```python
from build123d import *

# Parameters (mm, degrees)
SKETCH1_R         = 15
BODY_DEPTH        = 7
SKETCH2_R         = 11.5
CENTER_HOLE_DEPTH = 18
SKETCH4_W         = 4
SKETCH4_H         = 18.83157123
HEX_2_DEPTH       = 4


with BuildPart() as part:
    # Sketch1 → Body (new body)
    with BuildSketch(Plane(origin=(0, 0, 0), x_dir=(1, 0, 0), z_dir=(0, 1, 0))):
        Circle(SKETCH1_R)
    extrude(amount=BODY_DEPTH)

    # Sketch2 → Center_hole (cut)
    with BuildSketch(Plane(origin=(0, 7, 0), x_dir=(1, 0, 0), z_dir=(0, 1, 0))):
        Circle(SKETCH2_R)
    extrude(amount=-CENTER_HOLE_DEPTH, mode=Mode.SUBTRACT)

    # Sketch4 → Hex 2 (cut)
    with BuildSketch(Plane(origin=(0, 7, 0), x_dir=(1, 0, 0), z_dir=(0, 1, 0))):
        with Locations((15, 0)):
            Rectangle(SKETCH4_W, SKETCH4_H)
        with Locations((-15, 0)):
            Rectangle(SKETCH4_W, SKETCH4_H)
    extrude(amount=-HEX_2_DEPTH, mode=Mode.SUBTRACT)


solid = part.part
```
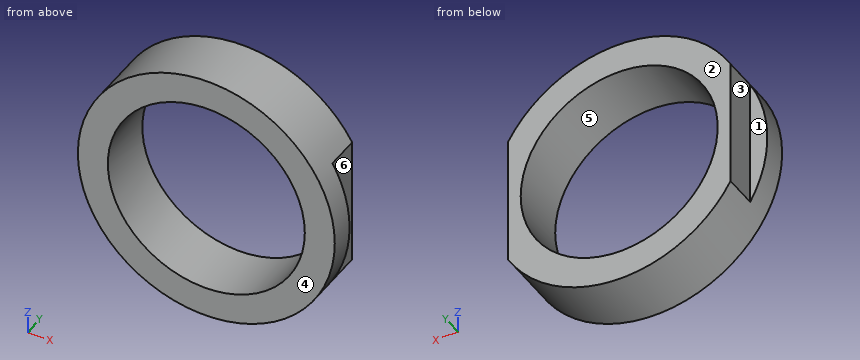
CAD build for the part. Positions are in the model's coordinates, mm. Face numbers are marked on the shaded views. A direction names the side the tool comes from. Round coordinates to 2 decimals unless told otherwise and drop trailing zeros. Order: outer loops, then holes, each group sorted by start corner. A loop starts at its lowest first (then second) coordinate and runs counter-clockwise, first axis right, second up.
Q1. Which spindle directions (+Z, -Z, +X, -X, +Y, -Y) get a long thin tool onto all of the face, cutting with end or side? Do the marked faces 1 and 2. Say none if no direction does.
Q2. Slice it at A-A (x = 0). Write the cut outline in (y, z), and give its area (3 significant figures).
Q3. Slice it at C-C (y = 2). Write the cut outline in (x, z), and give its area (3 significant figures).
Q4. Two-plate mould, pull along X, no slides. Class the marked faces 3, 4, 5 and 6: pulls with the +X half, pulls with the -X half, needs draft (parallel to the pull), parting line crosses it, or undercut.
Q5. Wall check: L1, parallel to X at y = 2, z = 0; L2, parallel to X at y = 5.5, z = 0. Give the ranges that are in metal, low to high.
Q6. Slice it at D-D (x = -7.75). Write the cut outline in (y, z), and give its area (3 significant figures).
Q7. Slice it at B-B (z = 0). Write the cut outline in (x, y).
Q8. Drop flat-ended pins along their axis: pin 1 (1.6 mm diameter, centred on x = 14, z = 3.5, fed in from +Y); pin 2 (1 mm diameter, centred on x = -1.5, y = 6, fed in from +Z); pin 3 (1.2 mm diameter, centred on y = 4.5, z = -2.5, fed in from -X). Give the stop position or say it passes through.
Results below:
1. face 1: +Z, -Z, -X, +Y
1. face 2: +Z, -Z, +X, -X, +Y
2. outline: (0, -15) - (7, -15) - (7, -11.5) - (0, -11.5) - close; (0, 11.5) - (7, 11.5) - (7, 15) - (0, 15) - close
2. area: 49.0 mm2
3. outline: circle Ø30 at (0, 0); hole circle Ø23 at (0, 0)
3. area: 291 mm2
4. face 3: pulls with the -X half
4. face 4: needs draft
4. face 5: undercut
4. face 6: pulls with the +X half
5. L1: x = -15 to -11.5, 11.5 to 15
5. L2: x = -13 to -11.5, 11.5 to 13
6. outline: (0, -12.84) - (7, -12.84) - (7, -8.5) - (0, -8.5) - close; (0, 8.5) - (7, 8.5) - (7, 12.84) - (0, 12.84) - close
6. area: 60.9 mm2
7. outline: (-15, 0) - (-11.5, 0) - (-11.5, 7) - (-13, 7) - (-13, 3) - (-15, 3) - close; (11.5, 0) - (15, 0) - (15, 3) - (13, 3) - (13, 7) - (11.5, 7) - close
8. pin 1: stops at y = 3
8. pin 2: stops at z = 14.97
8. pin 3: stops at x = -13
